```python
from build123d import *

# Parameters (mm, degrees)
SKETCH3_R               = 26
SKETCH3_R_2             = 24
BOSS_EXTRUDE1_DEPTH     = 82
SKETCH2_R               = 24.6
SKETCH2_R_2             = 22.6
BOSS_EXTRUDE2_DEPTH     = 30
CUT_EXTRUDE1_DEPTH      = 30
CUT_EXTRUDE1_DEPTH_BACK = 30
SKETCH5_W               = 101.816386604
SKETCH5_H               = 90.816460778
CUT_EXTRUDE2_DEPTH      = 30
SKETCH6_W               = 2
SKETCH6_H               = 20.775230247
BOSS_EXTRUDE3_DEPTH     = 61
BOSS_EXTRUDE5_DEPTH     = 25
CUT_EXTRUDE3_START      = -32
SKETCH8_R               = 22.6
CUT_EXTRUDE3_DEPTH      = 32


with BuildPart() as part:
    # Sketch3 → Boss-Extrude1 (new body)
    with BuildSketch(Plane(origin=(-103.870896529, 742.017814767, 0), x_dir=(-0.9903438719336157, -0.13863266326351154, 0), z_dir=(0.13863266326351156, -0.9903438719336158, 0))):
        with Locations(Location((-535.354479902, 0, 0), (0, 0, 180))):
            Circle(SKETCH3_R)
        with Locations(Location((-535.354479902, 0, 0), (0, 0, 180))):
            Circle(SKETCH3_R_2, mode=Mode.SUBTRACT)
    extrude(amount=-BOSS_EXTRUDE1_DEPTH)

    # Sketch4 → Cut-Extrude1 (cut, two sides: drawn at the far end of the back side and taken through both)
    with BuildSketch(Plane.XY.offset(-CUT_EXTRUDE1_DEPTH_BACK)):
        Polygon((414.924769966, 897.597101018), (426.314131953, 816.235432106), (452.063072624, 819.839881351), (440.673710637, 901.201550263), align=None)
    extrude(amount=CUT_EXTRUDE1_DEPTH + CUT_EXTRUDE1_DEPTH_BACK, mode=Mode.SUBTRACT)


with BuildPart() as body_2:
    # Sketch2 → Boss-Extrude2 (new body)
    with BuildSketch(Plane(origin=(455.481917253, 0, 0), x_dir=(0, 0, -1), z_dir=(1, 0, 0))):
        with Locations((0, 857.898759871)):
            Circle(SKETCH2_R)
        with Locations((0, 857.898759871)):
            Circle(SKETCH2_R_2, mode=Mode.SUBTRACT)
    extrude(amount=BOSS_EXTRUDE2_DEPTH)


with BuildPart() as cut_extrude2_tool:
    # Sketch5 → Cut-Extrude2 (new body)
    with BuildSketch(Plane.XY):
        with Locations((437.415428166, 854.729783017)):
            Rectangle(SKETCH5_W, SKETCH5_H)
    extrude(amount=-CUT_EXTRUDE2_DEPTH)


with BuildPart() as part_1:
    add(part.part)

    # Cut-Extrude2: cut by cut_extrude2_tool
    add(cut_extrude2_tool.part, mode=Mode.SUBTRACT)



with BuildPart() as body_2_1:
    add(body_2.part)

    # Cut-Extrude2: cut by cut_extrude2_tool
    add(cut_extrude2_tool.part, mode=Mode.SUBTRACT)


with BuildPart() as part_2:
    add(part_1.part)

    add(body_2_1.part)  # Boss-Extrude3 merges body 2
    # Sketch6 → Boss-Extrude3 (add)
    with BuildSketch(Plane(origin=(530.185028483, 74.217617339, 0), x_dir=(0, 0, -1), z_dir=(0.9903438719336157, 0.13863266326351165, 0))):
        with Locations((-25, 784.889811472)):
            Rectangle(SKETCH6_W, SKETCH6_H)
    extrude(amount=BOSS_EXTRUDE3_DEPTH)

    # Sketch7 → Boss-Extrude5 (add)
    with BuildSketch(Plane(origin=(590.596004671, 82.674209798, 0), x_dir=(0, 0, -1), z_dir=(0.9903438719336163, 0.1386326632635082, 0))):
        with BuildLine():
            Line((-26, 774.502196348), (-26, 795.277426595))
            Line((-26, 795.277426595), (-20.191250984, 795.277426595))
            ThreePointArc((-20.191250984, 795.277426595), (-24.123503055, 785.245711867), (-23.302052486, 774.502196348))
            Line((-23.302052486, 774.502196348), (-26, 774.502196348))
        make_face()
    extrude(amount=-BOSS_EXTRUDE5_DEPTH)

    # Sketch8 → Cut-Extrude3 (cut)
    with BuildSketch(Plane(origin=(485.481917253, 0, 0), x_dir=(0, 0, -1), z_dir=(1, 0, 0)).offset(CUT_EXTRUDE3_START)):
        with Locations((0, 857.898759871)):
            Circle(SKETCH8_R)
    extrude(amount=CUT_EXTRUDE3_DEPTH, mode=Mode.SUBTRACT)


solid = part_2.part
```
Geometry check sheet. Reference: the model listing, model coordinates, mm. A direction names the side the tool comes from. Give positions to 0.01 mm unless a question says otherwise; leave off trailing zeros. Write each loop counter-clockwise with the first axis right and the second up, starting at its lowest first coordinate (ties: lowest second). Pieces come first, ordered by that corner, then holes.
1) Release check for a two-part mould opening along Z. For faces 4 (the flat face through (396, 854, 0)), 5 (the cylindrical face through (470.8, 849.4, 23.7)), 6 (the cylindrical face through (402.704, 853.751, 18.586)), 7 (the flat face through (417.405, 879.879, 24.986)) record: pulls with the +Z half, pulls with the -Z half, needs draft (parallel to the pull), parting line crosses it, or undercut.
2) Section check C-C, the plane x = 452. Record the boundary of the cut face in (y, z).
3) Gauge pin test, flat ends, axial feed: pin 1 (1.5 mm diameter, centred on y = 845.5, z = 7, fed in from -X); pin 2 (10 mm diameter, centred on x = 447.5, z = 16, fed in from +Y); pin 3 (4 mm diameter, centred on y = 844, z = 20.5, fed in from -X); pin 4 (1.5 mm diameter, centred on x = 473.5, z = 20, fed in from -Y). Record the tip position at first contact, or that the pin passes through.
4) Access from +Z, -Z, +X, -X, +Y, -Y to the whole of each face (thin tool, end or side, straight path). Record for faces 1 (the cylindrical face through (404.089, 853.944, 17.156)), 2 (the flat face through (456.429, 866.924, 24.717)), 3 (the flat face through (424.54, 828.91, 24.99)).
5) Material ranges on L1, parallel to Y at x = 474.5, z = 5.5; L2, parallel to Z at x = 480.5, y = 861.5; L3, parallel to X at y = 864.5, z = 8.25, recorded low to high.
6) Section check A-A, the plane z = 15.5. Record the boundary of the cut face in (x, y).
7) Section check B-B, the plane z = 2.5. Record the boundary of the cut face in (x, y), and give its area (3 significant figures).
Computed:
1. face 4: pulls with the -Z half
1. face 5: undercut
1. face 6: pulls with the +Z half
1. face 7: needs draft
2. outline: (845.33, 24) - (866.3, 24) - (866.3, 26) - (845.33, 26) - close
3. pin 1: stops at x = 396.71
3. pin 2: passes through
3. pin 3: stops at x = 403.96
3. pin 4: stops at y = 842.58
4. face 1: -Z, +Y
4. face 2: +Z, +Y
4. face 3: +Z, -Z, +X
5. L1: y = 833.92 to 835.98, 879.82 to 881.88
5. L2: z = 22.31 to 26
5. L3: x = 394.66 to 396.8
6. outline: (394.27, 894.55) - (405.64, 813.34) - (408.17, 813.7) - (396.8, 894.9) - close; (455.48, 838.8) - (485.48, 838.8) - (485.48, 841.45) - (455.48, 841.45) - close; (455.48, 874.35) - (485.48, 874.35) - (485.48, 877) - (455.48, 877) - close
7. outline: (389.32, 893.86) - (400.68, 812.65) - (402.68, 812.93) - (391.31, 894.13) - close; (455.48, 833.43) - (485.48, 833.43) - (485.48, 835.44) - (455.48, 835.44) - close; (455.48, 880.36) - (485.48, 880.36) - (485.48, 882.37) - (455.48, 882.37) - close
7. area: 286 mm2
